```python
from build123d import *
from build123d.topology import SkipClean

# Parameters (mm, degrees)
SKETCH1_R           = 10.5
BOSS_EXTRUDE1_DEPTH = 22
SKETCH2_R           = 9.3
CUT_EXTRUDE1_DEPTH  = 3.75
BOSS_EXTRUDE3_START = 3.75
BOSS_EXTRUDE3_DEPTH = 3.75
CHAMFER1_SIZE       = 0.2
SKETCH4_W           = 6.6
SKETCH4_H           = 6.6
CUT_EXTRUDE2_DEPTH  = 24.527908959
CHAMFER2_SIZE       = 0.5
SKETCH6_R           = 5.5
CUT_EXTRUDE3_DEPTH  = 10


with BuildPart() as part:
    # Sketch1 → Boss-Extrude1 (new body)
    with BuildSketch(Plane.XY):
        Circle(SKETCH1_R)
    extrude(amount=BOSS_EXTRUDE1_DEPTH)

    # Sketch2 → Cut-Extrude1 (cut)
    with BuildSketch(Plane.XY.offset(22)):
        Circle(SKETCH2_R)
    extrude(amount=-CUT_EXTRUDE1_DEPTH, mode=Mode.SUBTRACT)

    # Sketch3 → Boss-Extrude3 (add)
    with BuildSketch(Plane.XY.offset(18.25).offset(BOSS_EXTRUDE3_START)):
        with BuildLine():
            Line((-1.45, 9.186266924), (-1.45, 7.186266924))
            Line((-1.45, 7.186266924), (1.45, 7.186266924))
            Line((1.45, 7.186266924), (1.45, 9.186266924))
            ThreePointArc((1.45, 9.186266924), (0, 9.3), (-1.45, 9.186266924))
        make_face()
        with BuildLine():
            Line((7.186266924, -1.45), (9.186266924, -1.45))
            ThreePointArc((9.186266924, -1.45), (9.3, 0), (9.186266924, 1.45))
            Line((9.186266924, 1.45), (7.186266924, 1.45))
            Line((7.186266924, 1.45), (7.186266924, -1.45))
        make_face()
        with BuildLine():
            Line((-1.45, -7.186266924), (-1.45, -9.186266924))
            ThreePointArc((-1.45, -9.186266924), (0, -9.3), (1.45, -9.186266924))
            Line((1.45, -9.186266924), (1.45, -7.186266924))
            Line((1.45, -7.186266924), (-1.45, -7.186266924))
        make_face()
        with BuildLine():
            Line((-7.186266924, 1.45), (-9.186266924, 1.45))
            ThreePointArc((-9.186266924, 1.45), (-9.3, 0), (-9.186266924, -1.45))
            Line((-9.186266924, -1.45), (-7.186266924, -1.45))
            Line((-7.186266924, -1.45), (-7.186266924, 1.45))
        make_face()
    extrude(amount=-BOSS_EXTRUDE3_DEPTH)

    # Chamfer1
    chamfer1_edges = [part.edges().sort_by_distance(p)[0] for p in [
        (-6.576093065, 6.576093065, 22),
        (1.45, 8.186266924, 22),
        (-1.45, 8.186266924, 22),
        (0, 7.186266924, 22),
        (6.576093065, 6.576093065, 22),
        (8.186266924, -1.45, 22),
        (8.186266924, 1.45, 22),
        (7.186266924, 0, 22),
        (6.576093065, -6.576093065, 22),
        (-1.45, -8.186266924, 22),
        (1.45, -8.186266924, 22),
        (0, -7.186266924, 22),
        (-6.576093065, -6.576093065, 22),
        (-8.186266924, 1.45, 22),
        (-8.186266924, -1.45, 22),
        (-7.186266924, 0, 22),
    ]]
    chamfer(chamfer1_edges, length=CHAMFER1_SIZE)

    # Sketch4 → Cut-Extrude2 (cut, through all)
    with BuildSketch(Plane.XY.offset(18.25)):
        Rectangle(SKETCH4_W, SKETCH4_H)
    extrude(amount=-CUT_EXTRUDE2_DEPTH, mode=Mode.SUBTRACT)

    # Chamfer2
    chamfer2_edges = [part.edges().sort_by_distance(p)[0] for p in [
        (3.3, 0, 0),
        (0, -3.3, 0),
        (-3.3, 0, 0),
        (0, 3.3, 0),
        (-10.5, 0, 0),
    ]]
    chamfer(chamfer2_edges, length=CHAMFER2_SIZE)

    # Sketch5 → Cut-Revolve1 (revolve, cut)
    with SkipClean():  # the faces are left unmerged after this step: merging them gives an invalid solid
        with BuildSketch(Plane(origin=(0, 0, 0), x_dir=(1, 0, 0), z_dir=(0, 1, 0))):
            with BuildLine():
                Line((3.3, -1.5), (3.3, -4.5))
                ThreePointArc((3.3, -4.5), (4.8, -3), (3.3, -1.5))
            make_face()
        revolve(axis=Axis((3.3, 0, 6.635415663), (0, 0, -1)), mode=Mode.SUBTRACT)

    # Sketch6 → Cut-Extrude3 (cut)
    with SkipClean():  # the faces are left unmerged after this step: merging them gives an invalid solid
        with BuildSketch(Plane.XY.offset(18.25)):
            Circle(SKETCH6_R)
        extrude(amount=-CUT_EXTRUDE3_DEPTH, mode=Mode.SUBTRACT)


solid = part.part
```
The model under review builds one solid part; all positions refer to its coordinate system, in mm. A direction names the side the tool comes from. Round coordinates to 2 decimals unless told otherwise and drop trailing zeros. Order: outer loops, then holes, each group sorted by start corner. A loop starts at its lowest first (then second) coordinate and runs counter-clockwise, first axis right, second up.
(1) Take a section at C-C, the plane z = 2.75. State the section outline as (x, y) points.
Working result:
outline: circle Ø21 at (0, 0); hole (-3.3, -3.3) - (3.3, -3.3) - (3.3, -1.48) arc R1.48 ccw to (3.3, 1.48) - (3.3, 3.3) - (-3.3, 3.3) - close
(2) For P1, Ø1, axis at x = 8, z = 19.5, coming from the -Y side; P2, Ø10, axis at x = -5, z = 7, coming from the +Y side; P3, Ø1, axis at x = -8, z = 20, coming from the +Y side; P4, Ø2, axis at x = 6.5, z = 19, coming from the +Y side, all flat-tipped, find the tip position at first contact; note any pin that passes through.
Working result:
P1: stops at y = -7.35
P2: stops at y = 10.5
P3: stops at y = 7.35
P4: stops at y = 8.94
(3) Take a section at D-D, the plane z = 13.25. State the section outline as (x, y) points, plus the area to 3 significant figures.
Working result:
outline: circle Ø21 at (0, 0); hole circle Ø11 at (0, 0)
area: 251 mm2
(4) Wall thickness on L1, parallel to Y at x = 0, z = 10.5; L2, parallel to Y at x = -0.25, z = 1.25; L3, parallel to Z at x = 2, y = 6.5: over which ranges is each line inside the solid? List them lowest first.
Working result:
L1: y = -10.5 to -5.5, 5.5 to 10.5
L2: y = -10.5 to -3.3, 3.3 to 10.5
L3: z = 0 to 18.25
(5) Take a section at B-B, the plane z = 7.25. State the section outline as (x, y) points.
Working result:
outline: circle Ø21 at (0, 0); hole (-3.3, -3.3) - (3.3, -3.3) - (3.3, 3.3) - (-3.3, 3.3) - close
(6) Tool access review of faces 1 (the face through (1.45, 8, 20)), 2 (the face through (0, 3.3, 4)): name each direction out of +Z, -Z, +X, -X, +Y, -Y from which nothing blocks a thin tool from reaching the whole face with its end or side.
Working result:
face 1: +Z
face 2: +Z, -Z
(7) Take a section at A-A, the plane x = 0. State the section outline as (y, z) points, plus the area to 3 significant figures.
Working result:
outline: (-10.5, 0.5) - (-10, 0) - (-3.8, 0) - (-3.3, 0.5) - (-3.3, 8.25) - (-5.5, 8.25) - (-5.5, 18.25) - (-7.19, 18.25) - (-7.19, 21.8) - (-7.39, 22) - (-10.5, 22) - close; (3.3, 0.5) - (3.8, 0) - (10, 0) - (10.5, 0.5) - (10.5, 22) - (7.39, 22) - (7.19, 21.8) - (7.19, 18.25) - (5.5, 18.25) - (5.5, 8.25) - (3.3, 8.25) - close
area: 243 mm2
(8) Mouldability with a two-part tool opening along Y and no side actions: class faces 3 (the face through (10, 3.2, 11.1)), 4 (the face through (-1.19, -5.37, 13.32)), 5 (the face through (-1, -8, 22)) as released by +Y, released by -Y, zero draft, split by the parting line, or undercut.
Working result:
face 3: split by the parting line
face 4: undercut
face 5: zero draft
